Input: part model. Units: mm. Frame: model coordinates. A direction names the side the tool comes from. Coordinates: 2 decimals unless noted, no trailing zeros. Loops run counter-clockwise (first coordinate to the right, second up) from the corner with the lowest first, then second, coordinate; pieces in that order, holes last. Notation, with made-up numbers: (76, 52) - (89, 52) arc R23 ccw to (89, 72) - close; hole circle Ø9 at (76, 3.25). An arc over 180 degrees is marked (long way). Use one line per item in the form item = value.
from build123d import *
from build123d.topology import SkipClean

# Parameters (mm, degrees)
SKETCH4_R              = 10.5
CUT_EXTRUDE2_DEPTH     = 2.75
SKETCH5_R              = 3.75
CUT_EXTRUDE3_DEPTH     = 0.7
SKETCH6_R              = 0.9
CUT_EXTRUDE4_DEPTH     = 50.775119287
SKETCH11_R             = 2
CUT_EXTRUDE8_DEPTH     = 50.70616159
CUT_EXTRUDE9_START     = -25
CUT_EXTRUDE9_OUTLINE_R = 1
CUT_EXTRUDE9_DEPTH     = 26
SKETCH18_R             = 30
CUT_EXTRUDE12_DEPTH    = 1
CUT_EXTRUDE13_START    = -1
SKETCH19_R             = 30
SKETCH19_R_2           = 15
CUT_EXTRUDE13_DEPTH    = 1
CUT_EXTRUDE14_DEPTH    = 50.989999
CIRPATTERN4_COUNT      = 5


with BuildPart() as part:
    # Sketch2 → Revolve1 (revolve)
    with BuildSketch(Plane(origin=(0, 0, 0), x_dir=(1, 0, 0), z_dir=(0, 1, 0))):
        Polygon((0, 0), (35, 0), (35, 2.5), (32, 2.5), (32, 5.5), (35, 5.5), (35, 8), (0, 8), align=None)
    revolve(axis=Axis((0, 0, 27.772111005), (0, 0, -1)))

    # Sketch4 → Cut-Extrude2 (cut)
    with BuildSketch(Plane.XY):
        Circle(SKETCH4_R)
    extrude(amount=-CUT_EXTRUDE2_DEPTH, mode=Mode.SUBTRACT)

    # Sketch5 → Cut-Extrude3 (cut)
    with BuildSketch(Plane.XY.offset(-2.75)):
        Circle(SKETCH5_R)
    extrude(amount=-CUT_EXTRUDE3_DEPTH, mode=Mode.SUBTRACT)

    # Sketch6 → Cut-Extrude4 (cut, through all)
    with BuildSketch(Plane.XY.offset(-2.75)):
        with Locations((0, 7)):
            Circle(SKETCH6_R)
        with Locations((4.949747468, 4.949747468)):
            Circle(SKETCH6_R)
        with Locations((7, 0)):
            Circle(SKETCH6_R)
        with Locations((4.949747468, -4.949747468)):
            Circle(SKETCH6_R)
        with Locations((0, -7)):
            Circle(SKETCH6_R)
        with Locations((-4.949747468, -4.949747468)):
            Circle(SKETCH6_R)
        with Locations((-7, 0)):
            Circle(SKETCH6_R)
        with Locations((-4.949747468, 4.949747468)):
            Circle(SKETCH6_R)
    extrude(amount=-CUT_EXTRUDE4_DEPTH, mode=Mode.SUBTRACT)

    # Sketch11 → Cut-Extrude8 (cut, through all)
    with BuildSketch(Plane.XY.offset(-3.45)):
        Circle(SKETCH11_R)
    extrude(amount=-CUT_EXTRUDE8_DEPTH, mode=Mode.SUBTRACT)

    # Cut-Extrude9: read off the stored shape, not the designer's step
    # Cut-Extrude9 outline → Cut-Extrude9 (cut)
    with BuildSketch(Plane(origin=(0, 32, 0), x_dir=(1, 0, 0), z_dir=(0, 1, 0)).offset(CUT_EXTRUDE9_START)):
        with Locations((0, 4.5)):
            Circle(CUT_EXTRUDE9_OUTLINE_R)
    extrude(amount=CUT_EXTRUDE9_DEPTH, mode=Mode.SUBTRACT)

    # Fillet4: read off the stored shape, not the designer's step
    # Fillet4 outline → Fillet4 (revolve, cut)
    with SkipClean():  # the faces are left unmerged after this step: merging them gives an invalid solid
        with BuildSketch(Plane.XZ.offset(-7)):
            with BuildLine():
                Line((1, -5.5), (1, -3.5))
                ThreePointArc((1, -3.5), (0.926138721, -3.398867689), (0.9, -3.276393202))
                Line((0.9, -3.276393202), (0.9, -5.723606798))
                ThreePointArc((0.9, -5.723606798), (0.926138721, -5.601132311), (1, -5.5))
            make_face()
        revolve(axis=Axis((0, 7, 0), (0, 0, 1)), mode=Mode.SUBTRACT)

    # Sketch18 → Cut-Extrude12 (cut)
    with SkipClean():  # the faces are left unmerged after this step: merging them gives an invalid solid
        with BuildSketch(Plane(origin=(0, 0, -8), x_dir=(-1, 0, 0), z_dir=(0, 0, -1))):
            Circle(SKETCH18_R)
        extrude(amount=-CUT_EXTRUDE12_DEPTH, mode=Mode.SUBTRACT)

    # Sketch19 → Cut-Extrude13 (cut)
    with SkipClean():  # the faces are left unmerged after this step: merging them gives an invalid solid
        with BuildSketch(Plane.XY.offset(CUT_EXTRUDE13_START)):
            with Locations(Location((0, 0, 0), (0, 0, 180))):
                Circle(SKETCH19_R)
            Circle(SKETCH19_R_2, mode=Mode.SUBTRACT)
        extrude(amount=CUT_EXTRUDE13_DEPTH, mode=Mode.SUBTRACT)

    # Sketch20 → Cut-Extrude14 (cut, symmetric)
    with SkipClean():  # the faces are left unmerged after this step: merging them gives an invalid solid
        with BuildSketch(Plane.XY.offset(-1)):
            with BuildLine():
                Line((12.435563588, 8.387893552), (21.991893156, 11.492933252))
                ThreePointArc((21.991893156, 11.492933252), (22.615992604, 12.084415431), (22.550191208, 12.941749359))
                ThreePointArc((22.550191208, 12.941749359), (15.28241656, 21.034441854), (5.339942751, 25.445726781))
                ThreePointArc((5.339942751, 25.445726781), (4.504235982, 25.243376874), (4.134560337, 24.467044982))
                Line((4.134560337, 24.467044982), (4.134560337, 14.418925439))
                ThreePointArc((4.134560337, 14.418925439), (8.816778784, 12.135254916), (12.435563588, 8.387893552))
            make_face()
        cut_extrude14 = extrude(amount=CUT_EXTRUDE14_DEPTH, both=True, mode=Mode.SUBTRACT)

    # CirPattern4: Cut-Extrude14 ×5 about axis
    with SkipClean():  # the faces are left unmerged after this step: merging them gives an invalid solid
        cirpattern4_axis = Axis((0, 0, 0), (0, 0, 1))
        for i in range(1, CIRPATTERN4_COUNT):
            add(cut_extrude14.rotate(cirpattern4_axis, i * 360 / CIRPATTERN4_COUNT), mode=Mode.SUBTRACT)


solid = part.part
Q1. Set-up query: faces 5 (the cylindrical face through (-6.94, 31.24, -4.02)), 6 (the cylindrical face through (-16.128, -25.296, -0.507)), 7 (the cylindrical face through (-15.158, 21.124, -3.958)). Return all of +Z, -Z, +X, -X, +Y, -Y with unobstructed straight access to the full face (end or side cutting, diameter ignored); none if empty.
Check values:
face_5 = none
face_6 = +Z
face_7 = +Z, -Z
Q2. First-contact query: P1, Ø8, axis at x = 5, y = -1, coming from the -Z side; P2, Ø1, axis at y = -6, z = -4, coming from the -X side; P3, Ø1, axis at y = -14.5, z = -6, coming from the +X side. Flat tips, straight axial feed; report the tip coordinate or a pass-through.
Check values:
P1 = -7
P2 = -31.52
P3 = 32.08
Q3. Cut plane C-C, the plane x = 29. Return loops of the section in (y, z), then the cut area to 3 significant figures.
Check values:
outline = (-19.6, -8) - (-7.68, -8) - (-7.68, -7) - (7.68, -7) - (7.68, -8) - (19.6, -8) - (19.6, -5.5) - (13.53, -5.5) - (13.53, -2.5) - (19.6, -2.5) - (19.6, 0) - (7.68, 0) - (7.68, -1) - (-7.68, -1) - (-7.68, 0) - (-19.6, 0) - (-19.6, -2.5) - (-13.53, -2.5) - (-13.53, -5.5) - (-19.6, -5.5) - close
area = 246 mm²
Q4. Cut plane A-A, the plane y = 23. Give the number of separate pieces and of enclosed holes in the cut face, then the cut area to 3 significant figures.
Check values:
separate_pieces = 3
enclosed_holes = 1
area = 221 mm²
Q5. Ray query, line 1 along Z through (x, y) = (12.5, 30); line 2 along X through (y, z) = (-8.5, -3.75); line 3 along X through (y, z) = (-4, -1.5). Return the intervals inside material, ascending. Write a range as [from, to].
Check values:
line_1 = [-8, -5.5], [-2.5, 0]
line_2 = [-30.85, -24.57], [-12.36, 12.36], [24.57, 30.85]
line_3 = [-34.77, -25.69], [-14.46, -9.71], [9.71, 14.46], [25.69, 34.77]
Q6. Pull-direction query (Y, two-part tool) for faces 1 (the cylindrical face through (10, 3.2, -1.4)), 2 (the cylindrical face through (-28, 21, -1)), 3 (the flat face through (-26, -16, 0)), 4 (the cylindrical face through (-18.494, -17.775, -3.958)); classes: pulls with the +Y half, pulls with the -Y half, needs draft (parallel to the pull), parting line crosses it, or undercut.
Check values:
face_1 = undercut
face_2 = parting line crosses it
face_3 = needs draft
face_4 = undercut
